Study the drawing (mm; zero at the part's minimum x, y, z) and answer. A direction names the side the tool comes from. Give positions to 0.01 mm unless a question says otherwise; leave off trailing zeros. Order: outer loops, then holes, each group sorted by start corner. A loop starts at its lowest first (then second) coordinate and runs counter-clockwise, first axis right, second up.
Item 1: A cutting plane is placed at A-A (z = 12.5). Write down the section's boundary in (x, y).
Item 2: Given pin 1 Ø12.5 at (x, z) = (15.5, 10.5) entering from -Y; pin 2 Ø2.5 at (x, y) = (11.5, 1.5) entering from -Z; pin 3 Ø1.5 at (y, z) = (1.5, 12) entering from +X; pin 4 Ø1.5 at (x, y) = (9.5, 9.5) entering from -Z, each flat-ended and moving along its own axis, determine where each tip first touches the part or whether it passes through.
Item 3: A cutting plane is placed at C-C (y = 6). Write down the section's boundary in (x, z).
Item 4: A cutting plane is placed at B-B (y = 10.5). Write down the section's boundary in (x, z).
Item 5: Which of the six approach directions +Z, -Z, +X, -X, +Y, -Y give full straight-line access (tool end or side, diameter ignored) to the marked faces 1, 2, 3, 4 and 5?
Item 6: A cutting plane is placed at D-D (y = 2.5). Write down the section's boundary in (x, z).
Item 7: The mould has two halves that part along Z. Classify the marked faces 6, 7 and 8: +Z half, -Z half, draft (parallel to the pull), parting line (faces both ways), or undercut.
Item 8: Find the intervals of material crossed by line 1 along Z through (x, y) = (12.5, 6.5); line 2 along X through (y, z) = (1.75, 12.5), in increasing order.
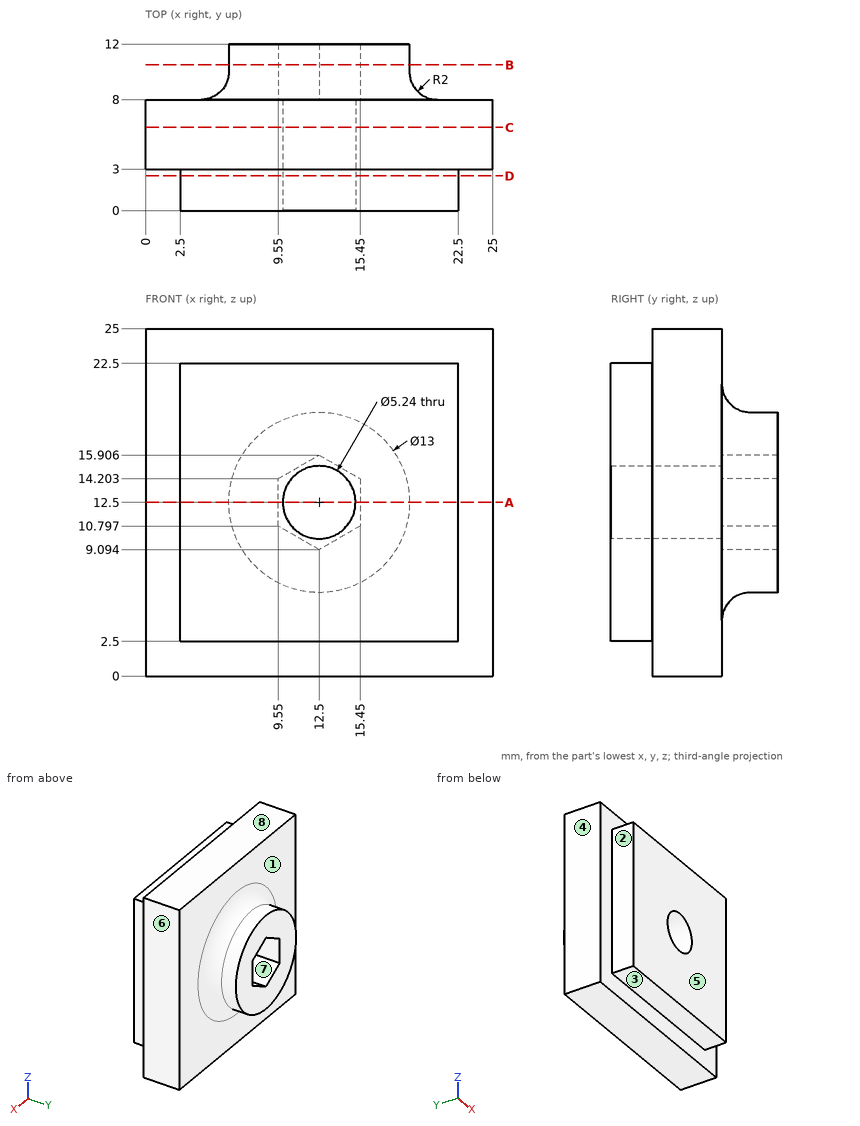
Response values:
1. outline: (0, 3) - (2.5, 3) - (2.5, 0) - (9.88, 0) - (9.88, 8) - (9.55, 8) - (9.55, 12) - (6, 12) - (6, 10) arc R2 cw to (4, 8) - (0, 8) - close; (15.12, 0) - (22.5, 0) - (22.5, 3) - (25, 3) - (25, 8) - (21, 8) arc R2 cw to (19, 10) - (19, 12) - (15.45, 12) - (15.45, 8) - (15.12, 8) - close
2. pin 1: stops at y = 0
2. pin 2: stops at z = 2.5
2. pin 3: stops at x = 22.5
2. pin 4: stops at z = 6.16
3. outline: (0, 0) - (25, 0) - (25, 25) - (0, 25) - close; hole circle Ø5.24 at (12.5, 12.5)
4. outline: circle Ø13 at (12.5, 12.5); hole (9.55, 10.8) - (12.5, 9.09) - (15.45, 10.8) - (15.45, 14.2) - (12.5, 15.91) - (9.55, 14.2) - close
5. face 1: +Y
5. face 2: +Z, -Z, -X, -Y
5. face 3: -Z, +X, -X, -Y
5. face 4: +Z, -Z, -X, +Y, -Y
5. face 5: +Z, -Z, +X, -X, -Y
6. outline: (2.5, 2.5) - (22.5, 2.5) - (22.5, 22.5) - (2.5, 22.5) - close; hole circle Ø5.24 at (12.5, 12.5)
7. face 6: draft
7. face 7: undercut
7. face 8: +Z half
8. line 1: z = 0 to 9.88, 15.12 to 25
8. line 2: x = 2.5 to 9.88, 15.12 to 22.5
